Geometry check sheet. Reference: the model listing, model coordinates, mm. A direction names the side the tool comes from. Coordinates: 2 decimals unless noted, no trailing zeros. Order: outer loops, then holes, each group sorted by start corner. A loop starts at its lowest first (then second) coordinate and runs counter-clockwise, first axis right, second up. Notation, with made-up numbers: M -6,-22 L 11,-22 A6 cw 11,-14 Z; hole C 67,-36.75 d9. An arc over 180 degrees is marked long. One line per item, written item: value. Start each with the question number.
1) Sectioned sample at B-B, the plane x = -16.25. Enter the section's corners in (y, z) (1 decimal), then the cut area to 3 significant figures.
2) Thickness scan on L1, parallel to X at y = 3.25, z = 0; L2, parallel to Z at x = -14, y = -0.25; L3, parallel to Z at x = -16.5, y = -3 (1 decimal). Record the ranges inside material, lowest first. Write a range as from..to.
3) Sectioned sample at C-C, the plane z = 0. State how many separate pieces and enclosed holes the cut face has, then the cut area to 3 significant figures.
4) Access from +Z, -Z, +X, -X, +Y, -Y to the whole of each face (thin tool, end or side, straight path). Record for faces 5 (the flat face through (-10, -3, -0.635)), 6 (the flat face through (-18, 2.54, 0)), 7 (the cylindrical face through (-20.42, 5.003, 0.088)).
5) Go/stop test with flat-tipped pins: P1, Ø3.5, axis at x = -11.5, y = -1, coming from the -Z side; P2, Ø4, axis at x = -4, y = -1, coming from the +Z side; P3, Ø3.5, axis at x = -14.27, z = 0, coming from the +Y side. Record where each tip stops, or that it passes through.
6) Draft check along X on faces 1 (the flat face through (-20, 1.575, 3)), 2 (the cylindrical face through (-6.603, 2.708, -0.174)), 3 (the conical face through (-16.968, 4.578, 0.764)), 4 (the flat face through (-21.234, 3, 0)). Enter one of: pulls with the +X half, pulls with the -X half, needs draft (parallel to the pull), parting line crosses it, or undercut.
```python
from build123d import *

# Parameters (mm, degrees)
SKETCH2_R           = 5.715
BOSS_EXTRUDE1_DEPTH = 18.9484
BOSS_EXTRUDE2_START = 2.286
BOSS_EXTRUDE2_DEPTH = 2.286
SKETCH6_W           = 0.635
SKETCH6_H           = 0.127
CUT_EXTRUDE2_DEPTH  = 1.778
CUT_EXTRUDE3_DEPTH  = 23.720523615
SKETCH12_R          = 1.3335
CUT_EXTRUDE4_DEPTH  = 6.096


with BuildPart() as part:
    # Sketch2 → Boss-Extrude1 (new body)
    with BuildSketch(Plane(origin=(0, 0, 0), x_dir=(0, 0, -1), z_dir=(1, 0, 0))):
        Circle(SKETCH2_R)
    extrude(amount=-BOSS_EXTRUDE1_DEPTH)

    # Sketch3 → Cut-Revolve1 (revolve, cut)
    with BuildSketch(Plane.XY, mode=Mode.PRIVATE) as cut_revolve1_sk:
        Polygon((-18.9484, 5.715), (-1.6764, 5.715), (-1.6764, 4.8895), (-2.794, 4.8895), (-2.794, 5.0038), (-15.9004, 5.0038), (-17.1704, 4.572), (-17.1704, 5.0038), (-18.9484, 5.0038), align=None)
    revolve(cut_revolve1_sk.sketch.rotate(Axis((0, 0, 0), (-1, 0, 0)), 90), axis=Axis((0, 0, 0), (-1, 0, 0)), mode=Mode.SUBTRACT)

    # Sketch5 → Boss-Extrude2 (add)
    with BuildSketch(Plane.ZY.offset(18.9484).offset(BOSS_EXTRUDE2_START)):
        with BuildLine():
            Line((-4.749528334, 1.5748), (4.749528334, 1.5748))
            ThreePointArc((4.749528334, 1.5748), (0, 5.0038), (-4.749528334, 1.5748))
        make_face()
    extrude(amount=-BOSS_EXTRUDE2_DEPTH)

    # Sketch6 → Cut-Revolve2 (revolve, cut)
    with BuildSketch(Plane.XY):
        with Locations((-19.2659, 4.9403)):
            Rectangle(SKETCH6_W, SKETCH6_H)
    revolve(axis=Axis((0, 0, 0), (1, 0, 0)), mode=Mode.SUBTRACT)

    # Sketch7 → Cut-Extrude2 (cut)
    with BuildSketch(Plane.ZY.offset(18.9484)):
        with BuildLine():
            Line((-2.484530314, -4.3434), (2.484530314, -4.3434))
            ThreePointArc((2.484530314, -4.3434), (0, -5.0038), (-2.484530314, -4.3434))
        make_face()
    extrude(amount=-CUT_EXTRUDE2_DEPTH, mode=Mode.SUBTRACT)

    # Sketch8 → Cut-Extrude3 (cut, through all)
    with BuildSketch(Plane(origin=(0, 0, 0), x_dir=(0, 0, -1), z_dir=(1, 0, 0))):
        Polygon((-0.635, -5.715), (1.8415, -5.715), (1.8415, -1.8395731), (0.635, -1.143), (0.635, 2.54), (-0.635, 2.54), (-0.635, -2.032), (0.635, -2.765234842), (0.635, -3.81), (-0.635, -3.81), align=None)
    extrude(amount=-CUT_EXTRUDE3_DEPTH, mode=Mode.SUBTRACT)

    # Sketch12 → Cut-Extrude4 (cut)
    with BuildSketch(Plane(origin=(0, 5.08, 0), x_dir=(1, 0, 0), z_dir=(0, 1, 0))):
        with Locations(Location((-4.7498, 0, 0), (0, 0, 270))):
            Circle(SKETCH12_R)
        with Locations(Location((-7.9248, 0, 0), (0, 0, 270))):
            Circle(SKETCH12_R)
        with Locations(Location((-11.0998, 0, 0), (0, 0, 270))):
            Circle(SKETCH12_R)
        with Locations(Location((-14.2748, 0, 0), (0, 0, 270))):
            Circle(SKETCH12_R)
    extrude(amount=-CUT_EXTRUDE4_DEPTH, mode=Mode.SUBTRACT)

    # Sketch13 → Cut-Revolve3 (revolve, cut)
    with BuildSketch(Plane.XY):
        with BuildLine():
            Line((0, 2.286), (0, -1.143))
            Line((0, -1.143), (-1.524, -1.143))
            ThreePointArc((-1.524, -1.143), (-1.180835312, 0.757649028), (0, 2.286))
        make_face()
    revolve(axis=Axis((-1.524, -1.143, 0), (1, 0, 0)), mode=Mode.SUBTRACT)


solid = part.part
```
Final values:
1. outline: M -4.8,0.6 L -3.8,0.6 L -3.8,-0.6 L -2.8,-0.6 L -2,0.6 L 2.5,0.6 L 2.5,-0.6 L -1.1,-0.6 L -1.8,-1.8 L -4.5,-1.8 A4.9 ccw long Z
1. area: 63.5 mm^2
2. L1: x = -21.23..-15.61, -12.94..-12.43, -9.77..-9.26, -6.59..-6.08, -3.42..0
2. L2: z = -5..-1.3, 1.3..5
2. L3: z = -3.7..-1.8, -0.6..3.7
3. separate pieces: 6
3. enclosed holes: 0
3. area: 51.9 mm^2
4. face 5: +X, -X, -Y
4. face 6: +X, -X
4. face 7: -X, +Y
5. P1: stops at z = -5
5. P2: stops at z = 5
5. P3: stops at y = 5
6. face 1: needs draft
6. face 2: undercut
6. face 3: undercut
6. face 4: pulls with the -X half
